Source: CAD feature listing. Evaluate the final solid. Frame: model axes, mm. A direction names the side the tool comes from. Coordinates: 2 decimals unless noted, no trailing zeros. Order: outer loops, then holes, each group sorted by start corner. A loop starts at its lowest first (then second) coordinate and runs counter-clockwise, first axis right, second up.
```python
from build123d import *

# Parameters (mm, degrees)
BOSS_EXTRUDE1_DEPTH = 6.35
CHAMFER1_SIZE       = 0.79375
SKETCH16_W          = 3.558466008
SKETCH16_H          = 3.18996611
CUT_EXTRUDE14_DEPTH = 208.663320883


# Read off the part's stored shape, not the designer's step: Boss-Extrude1
with BuildPart() as part:
    # Boss-Extrude1 outline → Boss-Extrude1 (new body)
    with BuildSketch(Plane.XY):
        with BuildLine():
            Line((22.436796564, 150), (19.069200519, 150))
            ThreePointArc((19.069200519, 150), (17.946668504, 150), (17.946668504, 151.122532015))
            Line((17.946668504, 151.122532015), (17.946668504, 158.877467985))
            ThreePointArc((17.946668504, 158.877467985), (17.946668504, 160), (19.069200519, 160))
            Line((19.069200519, 160), (22.436796564, 160))
            Line((22.436796564, 160), (22.436796564, 170))
            Line((22.436796564, 170), (19.069200519, 170))
            ThreePointArc((19.069200519, 170), (17.946668504, 170), (17.946668504, 171.122532015))
            Line((17.946668504, 171.122532015), (17.946668504, 178.877467985))
            ThreePointArc((17.946668504, 178.877467985), (17.946668504, 180), (19.069200519, 180))
            Line((19.069200519, 180), (22.436796564, 180))
            Line((22.436796564, 180), (22.436796564, 206.35))
            Line((22.436796564, 206.35), (17.436796564, 206.35))
            Line((17.436796564, 206.35), (17.436796564, 201.122532015))
            ThreePointArc((17.436796564, 201.122532015), (17.436796564, 200), (16.314264549, 200))
            Line((16.314264549, 200), (6.35, 200))
            Line((6.35, 200), (6.35, 191.122532015))
            ThreePointArc((6.35, 191.122532015), (6.35, 190), (5.227467985, 190))
            Line((5.227467985, 190), (0, 190))
            Line((0, 190), (0, 180))
            Line((0, 180), (5.227467985, 180))
            ThreePointArc((5.227467985, 180), (6.35, 180), (6.35, 178.877467985))
            Line((6.35, 178.877467985), (6.35, 171.122532015))
            ThreePointArc((6.35, 171.122532015), (6.35, 170), (5.227467985, 170))
            Line((5.227467985, 170), (0, 170))
            Line((0, 170), (0, 160))
            Line((0, 160), (5.227467985, 160))
            ThreePointArc((5.227467985, 160), (6.35, 160), (6.35, 158.877467985))
            Line((6.35, 158.877467985), (6.35, 151.122532015))
            ThreePointArc((6.35, 151.122532015), (6.35, 150), (5.227467985, 150))
            Line((5.227467985, 150), (0, 150))
            Line((0, 150), (0, 140))
            Line((0, 140), (5.227467985, 140))
            ThreePointArc((5.227467985, 140), (6.35, 140), (6.35, 138.877467985))
            Line((6.35, 138.877467985), (6.35, 131.122532015))
            ThreePointArc((6.35, 131.122532015), (6.35, 130), (5.227467985, 130))
            Line((5.227467985, 130), (0, 130))
            Line((0, 130), (0, 120))
            Line((0, 120), (5.227467985, 120))
            ThreePointArc((5.227467985, 120), (6.35, 120), (6.35, 118.877467985))
            Line((6.35, 118.877467985), (6.35, 111.122532015))
            ThreePointArc((6.35, 111.122532015), (6.35, 110), (5.227467985, 110))
            Line((5.227467985, 110), (0, 110))
            Line((0, 110), (0, 100))
            Line((0, 100), (5.227467985, 100))
            ThreePointArc((5.227467985, 100), (6.35, 100), (6.35, 98.877467985))
            Line((6.35, 98.877467985), (6.35, 91.122532015))
            ThreePointArc((6.35, 91.122532015), (6.35, 90), (5.227467985, 90))
            Line((5.227467985, 90), (0, 90))
            Line((0, 90), (0, 80))
            Line((0, 80), (5.227467985, 80))
            ThreePointArc((5.227467985, 80), (6.35, 80), (6.35, 78.877467985))
            Line((6.35, 78.877467985), (6.35, 71.122532015))
            ThreePointArc((6.35, 71.122532015), (6.35, 70), (5.227467985, 70))
            Line((5.227467985, 70), (0, 70))
            Line((0, 70), (0, 60))
            Line((0, 60), (5.227467985, 60))
            ThreePointArc((5.227467985, 60), (6.35, 60), (6.35, 58.877467985))
            Line((6.35, 58.877467985), (6.35, 51.122532015))
            ThreePointArc((6.35, 51.122532015), (6.35, 50), (5.227467985, 50))
            Line((5.227467985, 50), (0, 50))
            Line((0, 50), (0, 40))
            Line((0, 40), (5.227467985, 40))
            ThreePointArc((5.227467985, 40), (6.35, 40), (6.35, 38.877467985))
            Line((6.35, 38.877467985), (6.35, 31.122532015))
            ThreePointArc((6.35, 31.122532015), (6.35, 30), (5.227467985, 30))
            Line((5.227467985, 30), (0, 30))
            Line((0, 30), (0, 20))
            Line((0, 20), (5.227467985, 20))
            ThreePointArc((5.227467985, 20), (6.35, 20), (6.35, 18.877467985))
            Line((6.35, 18.877467985), (6.35, 11.122532015))
            ThreePointArc((6.35, 11.122532015), (6.35, 10), (5.227467985, 10))
            Line((5.227467985, 10), (0, 10))
            Line((0, 10), (0, 0))
            Line((0, 0), (16.314264549, 0))
            ThreePointArc((16.314264549, 0), (17.436796564, 0), (17.436796564, -1.122532015))
            Line((17.436796564, -1.122532015), (17.436796564, -6.35))
            Line((17.436796564, -6.35), (22.436796564, -6.35))
            Line((22.436796564, -6.35), (22.436796564, 10))
            Line((22.436796564, 10), (19.069200519, 10))
            ThreePointArc((19.069200519, 10), (17.946668504, 10), (17.946668504, 11.122532015))
            Line((17.946668504, 11.122532015), (17.946668504, 18.877467985))
            ThreePointArc((17.946668504, 18.877467985), (17.946668504, 20), (19.069200519, 20))
            Line((19.069200519, 20), (22.436796564, 20))
            Line((22.436796564, 20), (22.436796564, 30))
            Line((22.436796564, 30), (19.069200519, 30))
            ThreePointArc((19.069200519, 30), (17.946668504, 30), (17.946668504, 31.122532015))
            Line((17.946668504, 31.122532015), (17.946668504, 38.877467985))
            ThreePointArc((17.946668504, 38.877467985), (17.946668504, 40), (19.069200519, 40))
            Line((19.069200519, 40), (22.436796564, 40))
            Line((22.436796564, 40), (22.436796564, 50))
            Line((22.436796564, 50), (19.069200519, 50))
            ThreePointArc((19.069200519, 50), (17.946668504, 50), (17.946668504, 51.122532015))
            Line((17.946668504, 51.122532015), (17.946668504, 58.877467985))
            ThreePointArc((17.946668504, 58.877467985), (17.946668504, 60), (19.069200519, 60))
            Line((19.069200519, 60), (22.436796564, 60))
            Line((22.436796564, 60), (22.436796564, 70))
            Line((22.436796564, 70), (19.069200519, 70))
            ThreePointArc((19.069200519, 70), (17.946668504, 70), (17.946668504, 71.122532015))
            Line((17.946668504, 71.122532015), (17.946668504, 78.877467985))
            ThreePointArc((17.946668504, 78.877467985), (17.946668504, 80), (19.069200519, 80))
            Line((19.069200519, 80), (22.436796564, 80))
            Line((22.436796564, 80), (22.436796564, 90))
            Line((22.436796564, 90), (19.069200519, 90))
            ThreePointArc((19.069200519, 90), (17.946668504, 90), (17.946668504, 91.122532015))
            Line((17.946668504, 91.122532015), (17.946668504, 98.877467985))
            ThreePointArc((17.946668504, 98.877467985), (17.946668504, 100), (19.069200519, 100))
            Line((19.069200519, 100), (22.436796564, 100))
            Line((22.436796564, 100), (22.436796564, 110))
            Line((22.436796564, 110), (19.069200519, 110))
            ThreePointArc((19.069200519, 110), (17.946668504, 110), (17.946668504, 111.122532015))
            Line((17.946668504, 111.122532015), (17.946668504, 118.877467985))
            ThreePointArc((17.946668504, 118.877467985), (17.946668504, 120), (19.069200519, 120))
            Line((19.069200519, 120), (22.436796564, 120))
            Line((22.436796564, 120), (22.436796564, 130))
            Line((22.436796564, 130), (19.069200519, 130))
            ThreePointArc((19.069200519, 130), (17.946668504, 130), (17.946668504, 131.122532015))
            Line((17.946668504, 131.122532015), (17.946668504, 138.877467985))
            ThreePointArc((17.946668504, 138.877467985), (17.946668504, 140), (19.069200519, 140))
            Line((19.069200519, 140), (22.436796564, 140))
            Line((22.436796564, 140), (22.436796564, 150))
        make_face()
    extrude(amount=BOSS_EXTRUDE1_DEPTH)

    # Chamfer1
    chamfer1_edges = [part.edges().sort_by_distance(p)[0] for p in [
        (22.436796564, -6.35, 3.175),
        (17.436796564, -6.35, 3.175),
        (17.436796564, 206.35, 3.175),
        (22.436796564, 206.35, 3.175),
    ]]
    chamfer(chamfer1_edges, length=CHAMFER1_SIZE)

    # Sketch16 → Cut-Extrude14 (cut, through all)
    with BuildSketch(Plane.XZ):
        with Locations((13.182935446, 4.755016945)):
            Rectangle(SKETCH16_W, SKETCH16_H)
    extrude(amount=-CUT_EXTRUDE14_DEPTH, mode=Mode.SUBTRACT)


solid = part.part
```
1. Ray query, line 1 (X direction, y = 62.5, z = 5.25); line 2 (X direction, y = 119.5, z = 5.5); line 3 (X direction, y = 157, z = 2.25). Return the intervals inside material, ascending.
Findings:
line 1: x = 0 to 11.4, 14.96 to 22.44
line 2: x = 6.58 to 11.4, 14.96 to 17.72
line 3: x = 6.35 to 17.95
2. Section query A-A on y = 134. Return loops of the section in (x, z), plus the area to 3 significant figures.
Findings:
outline: (6.35, 0) - (17.95, 0) - (17.95, 6.35) - (14.96, 6.35) - (14.96, 3.16) - (11.4, 3.16) - (11.4, 6.35) - (6.35, 6.35) - close
area: 62.3 mm2
3. Access query for faces 4 (the face through (21, 50, 3)), 5 (the face through (6.35, 196, 3)), 6 (the face through (22.437, 145, 3)), 7 (the face through (3, 120, 3)). Directions: +Z, -Z, +X, -X, +Y, -Y. A direction counts if a zero-diameter tool reaches every point of the face in a straight line with its end or side. Return the directions, or none.
Findings:
face 4: +Z, -Z, +X
face 5: +Z, -Z, -X, +Y
face 6: +Z, -Z, +X, +Y, -Y
face 7: +Z, -Z, -X
4. Draft query along Y for faces 1 (the face through (20, 206.35, 3)), 2 (the face through (21, 110, 3)), 3 (the face through (0, 25, 3)). Return one class per face: released by +Y, released by -Y, zero draft, split by the parting line, or undercut.
Findings:
face 1: released by +Y
face 2: undercut
face 3: zero draft
5. Section query D-D on x = 9.5. Return loops of the section in (y, z), plus the area to 3 significant figures.
Findings:
outline: (0, 0) - (200, 0) - (200, 6.35) - (0, 6.35) - close
area: 1,270 mm2
6. Section query C-C on y = 24.5. Return loops of the section in (x, z).
Findings:
outline: (0, 0) - (22.44, 0) - (22.44, 6.35) - (14.96, 6.35) - (14.96, 3.16) - (11.4, 3.16) - (11.4, 6.35) - (0, 6.35) - close
7. Section query B-B on x = 1.75. Count the separate pieces of the cut face and the enclosed holes in it, plus the area to 3 significant figures.
Findings:
separate pieces: 10
enclosed holes: 0
area: 635 mm2
8. Pin query (flat end, axial travel): P1, Ø1.5, axis at x = 15.5, z = 3, coming from the +Y side; P2, Ø2.5, axis at x = 1.5, z = 4.5, coming from the +Y side; P3, Ø1.9, axis at y = 34, z = 4, coming from the +X side. Return the tip coordinate at first contact, or that it passes through.
Findings:
P1: stops at y = 200
P2: stops at y = 190
P3: stops at x = 17.95
